from build123d import *

# Parameters (mm, degrees)
F0_R     = 12.714699
F0_R_2   = 10.551867
F1_DEPTH = 6.35
F3_DEPTH = 6.35
F4_R     = 12.723011
F4_R_2   = 10.633663
F5_DEPTH = 6.35


with BuildPart() as f1:
    # F0 (on Top) → F1 (new body)
    with BuildSketch(Plane.XY):
        Circle(F0_R)
        Circle(F0_R_2, mode=Mode.SUBTRACT)
    extrude(amount=F1_DEPTH)

    # F2 (on Top) → F3 (join)
    with BuildSketch(Plane.XY):
        with BuildLine():
            ThreePointArc((4.443993, -26.840774), (1.994112, -19.590243), (3.689282, -12.127099))
            ThreePointArc((3.689282, -12.127099), (-0.691024, -12.712131), (-4.990178, -11.689086))
            ThreePointArc((-4.990178, -11.689086), (-3.674645, -19.507252), (-6.686923, -26.840774))
            ThreePointArc((-6.686923, -26.840774), (-1.121465, -25.492814), (4.443993, -26.840774))
        make_face()
    extrude(amount=F3_DEPTH)

    # F4 (on Top) → F5 (join)
    with BuildSketch(Plane.XY):
        with Locations((-2.609686, -37.986754)):
            Circle(F4_R)
        with Locations((-2.609686, -37.986754)):
            Circle(F4_R_2, mode=Mode.SUBTRACT)
    extrude(amount=F5_DEPTH)

    # F6: F1 across plane


with BuildPart() as f1_1:
    add(f1.part)
    add(f1.part.mirror(Plane.XZ))


solid = f1_1.part
Build history of the part. All positions in model axes, mm. Give positions to 0.01 mm unless a question says otherwise; leave off trailing zeros. Loops run counter-clockwise (first coordinate to the right, second up) from the corner with the lowest first, then second, coordinate; pieces in that order, holes last. Notation, with made-up numbers: (81, 71.5) - (113, 71.5) arc R13 cw to (113, 76.5) - close; hole circle Ø5 at (30, 42). An arc over 180 degrees is marked (long way). Write item = value, one per line. Start each with the question number.
1) Band-saw the part on B-B on z = 1.5. Give the cut face in (x, y), plus the area to 3 significant figures.
2) Band-saw the part on C-C on y = -33.5. Give the cut face in (x, z).
3) Probe probe 1 along Y at (x, z) = (7, 5.75); probe 2 along Y at (x, z) = (-5.5, 3.75); probe 3 along Y at (x, z) = (-11.5, 4.5). List the from-to ranges inside material, lowest first. Write a range as from..to.
4) Band-saw the part on D-D on y = -19.5. Give the cut face in (x, z).
5) Drop flat-ended pins along their axis: pin 1 Ø4 at (x, y) = (5.5, -40) entering from -Z; pin 2 Ø3 at (x, z) = (6.5, 4.5) entering from -Y. Give the stop position or say it passes through.
6) Band-saw the part on A-A on y = 0. Give the cut face in (x, z), plus the area to 3 significant figures.
7) Pull direction Y, two halves, no side cores. Call faces 1 (the cylindrical face through (-12.713, 0.208, 3.131)), 2 (the flat face through (-1, 11, 6.35)), 3 (the cylindrical face through (-3.607, 18.703, 3.131)): +Y half, -Y half, draft (parallel to the pull), parting line (faces both ways), or undercut.
Final values:
q1.outline = (-5.87, -25.69) arc R12.72 ccw (long way) to (0.09, -25.55) arc R12.16 cw to (4.44, -26.84) arc R14.11 cw to (3.66, -12.18) arc R12.71 ccw to (3.66, 12.18) arc R14.11 cw to (4.44, 26.84) arc R12.16 cw to (0.09, 25.55) arc R12.72 ccw (long way) to (-5.87, 25.69) arc R14.43 cw to (-4.99, 11.7) arc R12.71 ccw to (-4.99, -11.7) arc R14.43 cw to start; hole circle Ø21.27 at (-2.61, -37.99); hole circle Ø21.27 at (-2.61, 37.99); hole circle Ø21.1 at (0, 0); hole (-4.62, -11.84) arc R12.13 ccw to (1.36, -12.64) arc R12.71 cw to start; hole (-4.62, 11.84) arc R12.71 cw to (1.36, 12.64) arc R12.13 ccw to start
q1.area = 640 mm²
q2.outline = (-14.52, 0) - (-12.25, 0) - (-12.25, 6.35) - (-14.52, 6.35) - close; (7.03, 0) - (9.3, 0) - (9.3, 6.35) - (7.03, 6.35) - close
q3.probe_1 = -46.33..-42.54, -33.43..-29.65, -10.61..-7.9, 7.9..10.61, 29.65..33.43, 42.54..46.33
q3.probe_2 = -50.38..-48.22, -27.75..-25.09, -11.46..-9.01, 9.01..11.46, 25.09..27.75, 48.22..50.38
q3.probe_3 = -47.09..-43.82, -32.15..-28.89, -5.42..5.42, 28.89..32.15, 43.82..47.09
q4.outline = (-3.67, 0) - (1.99, 0) - (1.99, 6.35) - (-3.67, 6.35) - close
q5.pin_1 = through
q5.pin_2 = -48.18
q6.outline = (-12.71, 0) - (-10.55, 0) - (-10.55, 6.35) - (-12.71, 6.35) - close; (10.55, 0) - (12.71, 0) - (12.71, 6.35) - (10.55, 6.35) - close
q6.area = 27.5 mm²
q7.face_1 = undercut
q7.face_2 = draft
q7.face_3 = undercut
